from build123d import *

# Parameters (mm, degrees)
SKETCH1_W           = 80
SKETCH1_H           = 43
SKETCH1_R           = 3.5
SKETCH1_R_2         = 4.445
BOSS_EXTRUDE1_DEPTH = 18.5
SKETCH1_4_R         = 4.35
SKETCH1_4_R_2       = 3.5
CUT_EXTRUDE1_DEPTH  = 6
FILLET1_R           = 30
FILLET2_R           = 5
BOSS_EXTRUDE2_START = 18.5
SKETCH1_5_R         = 6
SKETCH1_5_R_2       = 4.445
BOSS_EXTRUDE2_DEPTH = 4.3864


with BuildPart() as part:
    # Sketch1 → Boss-Extrude1 (new body)
    with BuildSketch(Plane(origin=(0, 0, 0), x_dir=(1, 0, 0), z_dir=(0, 1, 0))):
        with Locations((40, -29.5)):
            Rectangle(SKETCH1_W, SKETCH1_H)
        with Locations(Location((26, -15, 0), (0, 0, 270))):
            Circle(SKETCH1_R, mode=Mode.SUBTRACT)
        with Locations(Location((54, -15, 0), (0, 0, 270))):
            Circle(SKETCH1_R, mode=Mode.SUBTRACT)
        with Locations(Location((26, -36, 0), (0, 0, 270))):
            Circle(SKETCH1_R, mode=Mode.SUBTRACT)
        with Locations(Location((54, -36, 0), (0, 0, 270))):
            Circle(SKETCH1_R, mode=Mode.SUBTRACT)
        with Locations(Location((70, -25.5, 0), (0, 0, 270))):
            Circle(SKETCH1_R_2, mode=Mode.SUBTRACT)
        with Locations(Location((10, -25.5, 0), (0, 0, 270))):
            Circle(SKETCH1_R_2, mode=Mode.SUBTRACT)
    extrude(amount=BOSS_EXTRUDE1_DEPTH)

    # Sketch1_4 → Cut-Extrude1 (cut)
    # profile 1 of 4: a face of its own
    with BuildSketch(Plane(origin=(0, 0, 0), x_dir=(1, 0, 0), z_dir=(0, 1, 0))):
        with Locations(Location((26, -15, 0), (0, 0, 270))):
            Circle(SKETCH1_4_R)
        with Locations(Location((26, -15, 0), (0, 0, 270))):
            Circle(SKETCH1_4_R_2, mode=Mode.SUBTRACT)
    # profile 2 of 4: a face of its own
    with BuildSketch(Plane(origin=(0, 0, 0), x_dir=(1, 0, 0), z_dir=(0, 1, 0))):
        with Locations(Location((54, -15, 0), (0, 0, 270))):
            Circle(SKETCH1_4_R)
        with Locations(Location((54, -15, 0), (0, 0, 270))):
            Circle(SKETCH1_4_R_2, mode=Mode.SUBTRACT)
    # profile 3 of 4: a face of its own
    with BuildSketch(Plane(origin=(0, 0, 0), x_dir=(1, 0, 0), z_dir=(0, 1, 0))):
        with Locations(Location((54, -36, 0), (0, 0, 270))):
            Circle(SKETCH1_4_R)
        with Locations(Location((54, -36, 0), (0, 0, 270))):
            Circle(SKETCH1_4_R_2, mode=Mode.SUBTRACT)
    # profile 4 of 4: a face of its own
    with BuildSketch(Plane(origin=(0, 0, 0), x_dir=(1, 0, 0), z_dir=(0, 1, 0))):
        with Locations(Location((26, -36, 0), (0, 0, 270))):
            Circle(SKETCH1_4_R)
        with Locations(Location((26, -36, 0), (0, 0, 270))):
            Circle(SKETCH1_4_R_2, mode=Mode.SUBTRACT)
    extrude(amount=CUT_EXTRUDE1_DEPTH, mode=Mode.SUBTRACT)

    # Fillet1
    fillet1_edges = [part.edges().sort_by_distance(p)[0] for p in [
        (80, 9.25, 51),
        (0, 9.25, 51),
    ]]
    fillet(fillet1_edges, radius=FILLET1_R)

    # Fillet2
    fillet2_edges = [part.edges().sort_by_distance(p)[0] for p in [
        (0, 9.25, 8),
        (80, 9.25, 8),
    ]]
    fillet(fillet2_edges, radius=FILLET2_R)

    # Sketch1_5 → Boss-Extrude2 (add)
    # profile 1 of 2: a face of its own
    with BuildSketch(Plane(origin=(0, 0, 0), x_dir=(1, 0, 0), z_dir=(0, 1, 0)).offset(BOSS_EXTRUDE2_START)):
        with Locations(Location((70, -25.5, 0), (0, 0, 270))):
            Circle(SKETCH1_5_R)
        with Locations(Location((70, -25.5, 0), (0, 0, 270))):
            Circle(SKETCH1_5_R_2, mode=Mode.SUBTRACT)
    # profile 2 of 2: a face of its own
    with BuildSketch(Plane(origin=(0, 0, 0), x_dir=(1, 0, 0), z_dir=(0, 1, 0)).offset(BOSS_EXTRUDE2_START)):
        with Locations(Location((10, -25.5, 0), (0, 0, 270))):
            Circle(SKETCH1_5_R)
        with Locations(Location((10, -25.5, 0), (0, 0, 270))):
            Circle(SKETCH1_5_R_2, mode=Mode.SUBTRACT)
    extrude(amount=BOSS_EXTRUDE2_DEPTH)


solid = part.part
Design review of the part built by this model. Coordinates are the model's own, in mm. A direction names the side the tool comes from. Coordinates: 2 decimals unless noted, no trailing zeros. Order: outer loops, then holes, each group sorted by start corner. A loop starts at its lowest first (then second) coordinate and runs counter-clockwise, first axis right, second up. Notation, with made-up numbers: (10.25, -15.75) -> (30.25, -15.75) arc R21 cw to (30.25, -4.75) -> close; hole circle Ø3 at (45, 3). An arc over 180 degrees is marked (long way). Use one line per item in the form item = value. Start each with the question number.
(1) For faces 1 (the cylindrical face through (22.14, 2.96, 17.01)), 2 (the cylindrical face through (6.057, 11.283, 27.551)), list the 3-axis set-ups (+Z, -Z, +X, -X, +Y, -Y) from which the entire face can be reached by the end or side of a thin tool; tool diameter is ignored.
(2) Add section D-D on y = 20.5. State the section outline as (x, z) points (3 decimals), plus the area to 3 significant figures.
(3) For probe 1 along X at (y, z) = (10.25, 15); probe 2 along X at (y, z) = (1.8, 15); probe 3 along Z at (x, y) = (68, 15.5), list the stretches that pass through material, from the lowest coordinate up.
(4) Add section B-B on y = 3. State the section outline as (x, z) points (3 decimals), plus the area to 3 significant figures.
(5) Insertion check: pin 1 (10 mm diameter, centred on x = 54, z = 15, fed in from +Y); pin 2 (4 mm diameter, centred on y = 8.5, z = 29.5, fed in from -X); pin 3 (4 mm diameter, centred on y = 10, z = 40, fed in from -X). Each pin has a flat end and moves straight along its axis. Give the tip position at first contact, or say it passes through.
(6) Add section A-A on z = 15. State the section outline as (x, y) points.
(7) The part is to be moulded in two halves that separate along X. For faces 3 (the cylindrical face through (8.555, 9.38, 41.979)), 4 (the flat face through (40, 9, 8)), 5 (the cylindrical face through (56.365, 12.162, 33.42)), 6 (the cylindrical face through (78, 9, 9)), say which applies: +X half, -X half, draft (parallel to the pull), parting line (faces both ways), or undercut.
(8) Add section C-C on x = 70. State the section outline as (y, z) points (3 decimals).
Answer block:
q1.face_1 = -Y
q1.face_2 = +Y, -Y
q2.outline = circle Ø12 at (10, 25.5); circle Ø12 at (70, 25.5); hole circle Ø8.89 at (10, 25.5); hole circle Ø8.89 at (70, 25.5)
q2.area = 102 mm²
q3.probe_1 = 0 to 22.5, 29.5 to 50.5, 57.5 to 80
q3.probe_2 = 0 to 21.65, 30.35 to 49.65, 58.35 to 80
q3.probe_3 = 8 to 21.53, 29.47 to 45
q4.outline = (0, 13) arc R5 ccw to (5, 8) -> (75, 8) arc R5 ccw to (80, 13) -> (80, 21) arc R30 ccw to (50, 51) -> (30, 51) arc R30 ccw to (0, 21) -> close; hole circle Ø8.89 at (10, 25.5); hole circle Ø8.7 at (26, 15); hole circle Ø8.7 at (26, 36); hole circle Ø8.7 at (54, 15); hole circle Ø8.7 at (54, 36); hole circle Ø8.89 at (70, 25.5)
q4.area = 2,680 mm²
q5.pin_1 = 18.5
q5.pin_2 = 0.71
q5.pin_3 = 5.28
q6.outline = (0, 0) -> (21.65, 0) -> (21.65, 6) -> (22.5, 6) -> (22.5, 18.5) -> (0, 18.5) -> close; (29.5, 6) -> (30.35, 6) -> (30.35, 0) -> (49.65, 0) -> (49.65, 6) -> (50.5, 6) -> (50.5, 18.5) -> (29.5, 18.5) -> close; (57.5, 6) -> (58.35, 6) -> (58.35, 0) -> (80, 0) -> (80, 18.5) -> (57.5, 18.5) -> close
q7.face_3 = -X half
q7.face_4 = draft
q7.face_5 = undercut
q7.face_6 = +X half
q8.outline = (0, 8) -> (18.5, 8) -> (18.5, 19.5) -> (22.886, 19.5) -> (22.886, 21.055) -> (0, 21.055) -> close; (0, 29.945) -> (22.886, 29.945) -> (22.886, 31.5) -> (18.5, 31.5) -> (18.5, 43.361) -> (0, 43.361) -> close
